Study the drawing (mm; zero at the part's minimum x, y, z) and answer. Give positions to 0.01 mm unless a question says otherwise; leave off trailing zeros. Order: outer loops, then holes, each group sorted by start corner. A loop starts at its lowest first (then second) coordinate and runs counter-clockwise, first axis right, second up. Notation, with made-up numbers: (7.25, 81) - (17.25, 81) arc R31 ccw to (17.25, 118) - close; hole circle Ø4 at (58, 39.25). An arc over 180 degrees is marked (long way). Write each question's results on one line, items separated by ' | '. Start each with the question number.
Q1. Find section A-A on x = 19.05. Give the vertices of the cut face in (y, z) (3 decimals), and give its area (3 significant figures).
Q2. For a pull along X with two mould halves and no side action, classify the marked faces 1, 2 and 3 as +X half, -X half, draft (parallel to the pull), parting line (faces both ways), or undercut.
Q3. Find the intervals of material crossed by line 1 along Y through (x, z) = (19.05, 0.55); line 2 along Y through (x, z) = (19.05, 26) (3 decimals), in increasing order. Write a range as from..to.
Q4. Find section D-D on z = 24.5. Give the vertices of the cut face in (x, y).
Q5. Flat-ended cylindrical pins translate along their axes: P1, Ø3, axis at x = 17.5, z = 21, coming from the -Y side; P2, Ø6, axis at x = 18.5, z = 17, coming from the +Y side; P3, Ø17.5, axis at x = 19.05, y = 19.05, coming from the -Z side; P4, Ø2, axis at y = 19.5, z = 5, coming from the +X side. Find the tip coordinate at first contact, or state that the pin passes through.
Q6. Find section C-C on z = 14. Give the vertices of the cut face in (x, y) (3 decimals), and give its area (3 significant figures).
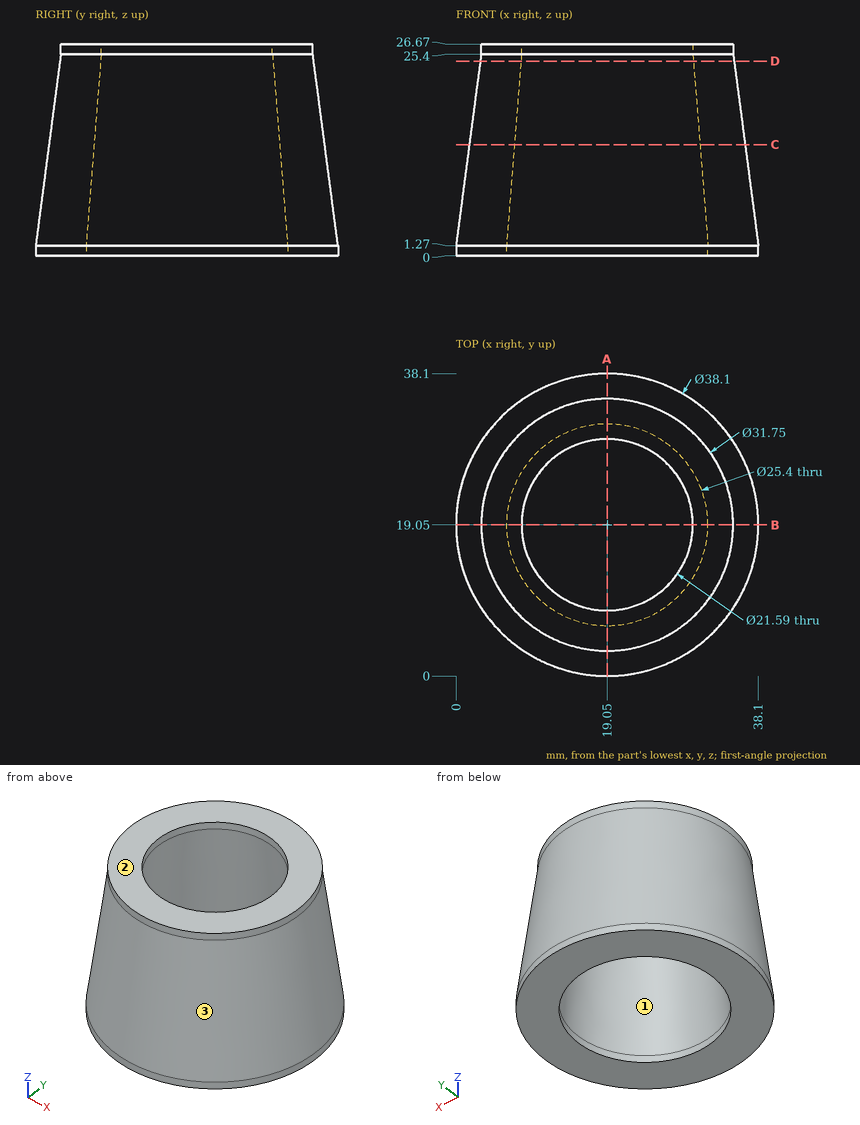
Working result:
1) outline: (0, 0) - (6.35, 0) - (6.35, 1.27) - (8.255, 25.4) - (8.255, 26.67) - (3.175, 26.67) - (3.175, 25.4) - (0, 1.27) - close; (29.845, 25.4) - (31.75, 1.27) - (31.75, 0) - (38.1, 0) - (38.1, 1.27) - (34.925, 25.4) - (34.925, 26.67) - (29.845, 26.67) - close | area: 305 mm²
2) face 1: undercut | face 2: draft | face 3: parting line
3) line 1: 0..6.35, 31.75..38.1 | line 2: 3.175..8.255, 29.845..34.925
4) outline: circle Ø31.99 at (19.05, 19.05); hole circle Ø21.73 at (19.05, 19.05)
5) P1: y = 2.44 | P2: y = 36.42 | P3: through | P4: x = 37.74
6) outline: circle Ø34.75 at (19.05, 19.05); hole circle Ø23.39 at (19.05, 19.05) | area: 519 mm²
